Work out the finished part from the listing and answer in its coordinate system (mm). Coordinates: 2 decimals unless noted, no trailing zeros. Loops run counter-clockwise (first coordinate to the right, second up) from the corner with the lowest first, then second, coordinate; pieces in that order, holes last. Notation, with made-up numbers: (-12.75, -28) - (-2.75, -28) arc R18 cw to (-2.75, -18) - close; hole circle Ø11 at (-39, -14). An arc over 180 degrees is marked (long way). Write each question's results on one line, items separated by ' | '. Start each with the question number.
Item 1: Consider probe 1 along Z at (x, y) = (-50, 0.9); probe 2 along Z at (x, y) = (-25.5, 2.75); probe 3 along X at (y, z) = (1.7, -0.5). Determine where each line is inside the solid, lowest interval first. Write a range as [from, to].
Item 2: Section B-B, the plane z = 0 is taken. Write down the section's boundary in (x, y).
Item 3: Section A-A, the plane y = 0.65 is taken. Write down the section's boundary in (x, z), plus the area to 3 significant figures.
Autodesk Inventor part; units mm, degrees
ref_plane "YZ Plane" through (0, 0, 0) normal (1, 0, 0) x (0, 1, 0)
ref_plane "XZ Plane" through (0, 0, 0) normal (0, 1, 0) x (-1, 0, 0)
ref_plane "XY Plane" through (0, 0, 0) normal (0, 0, 1) x (1, 0, 0)
sketch "Sketch1" plane through (0, 0, 0) normal (0, 1, 0) x (-1, 0, 0)
  line L0 (0, 0) -> (25, 0)
  line L1 (25, 0) -> (50, 0)
  circle A0 centre (50, 0) radius 2
  circle A1 centre (50, 0) radius 4
  circle A2 centre (0, 0) radius 4
  line L2 (0, 4) -> (50, 4)
  line L3 (0, -4) -> (50, -4)
  circle A3 centre (25, 0) radius 2.5
  line L4 (25, 0) -> (25, 1.5)
  line L5 (25, 1.5) -> (28.63, 1.5)
  line L6 (28.63, 1.5) -> (20.4744, 1.5)
  line L7 (20.4744, 1.5) -> (20.4744, -1.5)
  line L8 (20.4744, -1.5) -> (28.63, -1.5)
  line L9 (28.63, -1.5) -> (28.63, 1.5)
  circle A4 centre (0, 0) radius 2
  point P0 (27, 1.5)
  point P1 (27, -1.5)
  point P2 (23, -1.5)
  point P3 (23, 1.5)
  dimension "d1" = 25
  dimension "d2" = 25
  dimension "d3" = 4
  dimension "d4" = 8
  dimension "d5" = 8
  dimension "d6" = 5
  dimension "d7" = 1.5
  dimension "d8" = 3
  dimension "d9" = 4
extrude "Extrusion1" add sketch "Sketch1" along normal blind 3 contours A2 | A2 L2 A1 L1 L9 L5 A3 L6 L7 L0 | L0 L7 L8 A3 L9 L1 A1 L3 A2 | L7 L6 A3 L0 | L0 A3 L8 L7 | A1 | A3 L5 L6 | L8 A3 | A3 L5 L9 L1 | L1 L9 L8 A3
properties part number "stuurarm motor"
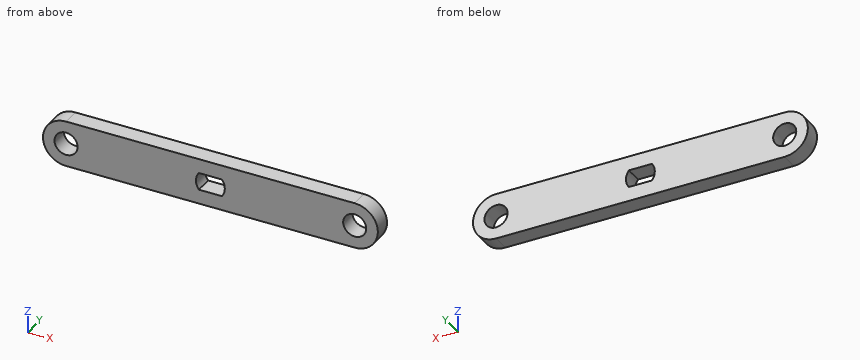
Answer key:
1) probe 1: z = [-4, -2], [2, 4] | probe 2: z = [-4, -1.5], [1.5, 4] | probe 3: x = [-53.97, -51.94], [-48.06, -27.45], [-22.55, -1.94], [1.94, 3.97]
2) outline: (-54, 0) - (-52, 0) - (-52, 3) - (-54, 3) - close; (-48, 0) - (-27.5, 0) - (-27.5, 3) - (-48, 3) - close; (-22.5, 0) - (-2, 0) - (-2, 3) - (-22.5, 3) - close; (2, 0) - (4, 0) - (4, 3) - (2, 3) - close
3) outline: (-50, -4) - (0, -4) arc R4 ccw to (0, 4) - (-50, 4) arc R4 ccw to start; hole circle Ø4 at (-50, 0); hole (-27, -1.5) - (-23, -1.5) arc R2.5 ccw to (-23, 1.5) - (-27, 1.5) arc R2.5 ccw to start; hole circle Ø4 at (0, 0) | area: 411 mm^2
